```python
from build123d import *

# Parameters (mm, degrees)
F0_R     = 101.6
F1_DEPTH = 76.2


with BuildPart() as f1:
    # F0 (on Front) → F1 (new body)
    with BuildSketch(Plane.XZ):
        with BuildLine():
            Line((-190.5, 1016), (-190.5, 0))
            ThreePointArc((-190.5, 0), (-134.703842, -134.703842), (0, -190.5))
            ThreePointArc((0, -190.5), (134.703842, -134.703842), (190.5, 0))
            Line((190.5, 0), (190.5, 1016))
            ThreePointArc((190.5, 1016), (134.703842, 1150.703842), (0, 1206.5))
            ThreePointArc((0, 1206.5), (-134.703842, 1150.703842), (-190.5, 1016))
        make_face()
        Circle(F0_R, mode=Mode.SUBTRACT)
        with Locations((0, 1016)):
            Circle(F0_R, mode=Mode.SUBTRACT)
    extrude(amount=F1_DEPTH)


solid = f1.part
```
Geometry: final body of the model. Coordinates: model frame, mm. Round coordinates to 2 decimals unless told otherwise and drop trailing zeros. Write each loop counter-clockwise with the first axis right and the second up, starting at its lowest first coordinate (ties: lowest second). Pieces come first, ordered by that corner, then holes.
Item 1: Section query D-D (x = 148). Return loops of the section in (y, z), plus the area to 3 significant figures.
Item 2: Section query A-A (y = -31). Return loops of the section in (x, z), plus the area to 3 significant figures.
Item 3: Section query B-B (z = 23.5). Return loops of the section in (x, y), plus the area to 3 significant figures.
Item 4: Material intervals for L1, parallel to Z at x = -5.5, y = -19; L2, parallel to Z at x = 0, y = -50; L3, parallel to X at y = -40, z = 1087.5, sorted ascending.
Item 5: Pin query (flat end, axial travel): P1, Ø2, axis at y = -67, z = 1022.5, coming from the +X side; P2, Ø2, axis at x = -93, y = -59, coming from the +Z side; P3, Ø10, axis at x = 84.5, y = -19.5, coming from the -Z side. Return the tip coordinate at first contact, or that it passes through.
Item 6: Section query C-C (x = -125). Return loops of the section in (y, z), plus the area to 3 significant figures.
Item 7: Mould query, pull axis Z, two halves, no side actions, for faces 1 (the face through (190.5, -38, 501)), 2 (the face through (-22.025, -37.567, -99.184)). Classes: +Z half, -Z half, draft (parallel to the pull), parting line (faces both ways), or undercut.
Completed:
1. outline: (-76.2, -119.94) - (0, -119.94) - (0, 1135.94) - (-76.2, 1135.94) - close
1. area: 95,700 mm2
2. outline: (-190.5, 0) arc R190.5 ccw to (0, -190.5) arc R190.5 ccw to (190.5, 0) - (190.5, 1016) arc R190.5 ccw to (0, 1206.5) arc R190.5 ccw to (-190.5, 1016) - close; hole circle Ø203.2 at (0, 0); hole circle Ø203.2 at (0, 1016)
2. area: 436,000 mm2
3. outline: (-190.5, -76.2) - (-98.84, -76.2) - (-98.84, 0) - (-190.5, 0) - close; (98.84, -76.2) - (190.5, -76.2) - (190.5, 0) - (98.84, 0) - close
3. area: 14,000 mm2
4. L1: z = -190.42 to -101.45, 101.45 to 914.55, 1117.45 to 1206.42
4. L2: z = -190.5 to -101.6, 101.6 to 914.4, 1117.6 to 1206.5
4. L3: x = -176.57 to -72.18, 72.18 to 176.57
5. P1: stops at x = 190.42
5. P2: stops at z = 1182.81
5. P3: stops at z = -173.12
6. outline: (-76.2, -143.75) - (0, -143.75) - (0, 1159.75) - (-76.2, 1159.75) - close
6. area: 99,300 mm2
7. face 1: draft
7. face 2: undercut
